from build123d import *

# Parameters (mm, degrees)
F0_W     = 50
F0_H     = 50
F1_DEPTH = 35
F3_DEPTH = 35.001
F5_DEPTH = 20


with BuildPart() as f1:
    # F0 (on Front) → F1 (new body)
    with BuildSketch(Plane.XZ):
        Rectangle(F0_W, F0_H)
    extrude(amount=F1_DEPTH)

    # F2 (on face) → F3 (cut, through all)
    with BuildSketch(Plane.XZ.offset(35)):
        Polygon((-25, 0), (18.30127, 25), (-25, 25), align=None)
    extrude(amount=-F3_DEPTH, mode=Mode.SUBTRACT)

    # F4 (on face) → F5 (cut)
    with BuildSketch(Plane.XZ.offset(35)):
        Polygon((-25, 0), (-25, -13), (25, -13), (25, 13), (-2.48334, 13), align=None)
    extrude(amount=-F5_DEPTH, mode=Mode.SUBTRACT)


solid = f1.part
Could you check a few things on this model? Use its own coordinates, in mm. A direction names the side the tool comes from. Give positions to 0.01 mm unless a question says otherwise; leave off trailing zeros. Write each loop counter-clockwise with the first axis right and the second up, starting at its lowest first coordinate (ties: lowest second). Pieces come first, ordered by that corner, then holes. Notation, with made-up numbers: (-3.75, 15.25) -> (26.25, 15.25) arc R5 ccw to (26.25, 21.25) -> close; hole circle Ø5 at (48.25, -30.5). An arc over 180 degrees is marked (long way). Write each question's results on one line, items separated by ' | '. Start each with the question number.
Q1. I'm going to push flat-ended pins straight in: pin 1 Ø2 at (x, y) = (-12.5, -31) entering from +Z; pin 2 Ø6 at (x, z) = (2.5, 4) entering from -Y; pin 3 Ø2 at (y, z) = (-20.5, 16.5) entering from -X. Where does each tip first touch, or does it pass through?
Q2. Suppose I cut it at A-A, the plane y = -20.5. List the corners of the cut face in (x, z) for me, and give its area (3 significant figures).
Q3. I need wall thicknesses on probe 1 along Z at (x, y) = (20, -18); probe 2 along Z at (x, y) = (-18.5, -27); probe 3 along Y at (x, z) = (19, 3). Which ranges of each line are inside material? Lowest first, please.
Q4. Suppose I cut it at D-D, the plane z = 21. List the corners of the cut face in (x, y) for me, and give its area (3 significant figures).
Q5. Suppose I cut it at C-C, the plane y = -11.5. List the corners of the cut face in (x, z) for me.
Q6. Suppose I cut it at B-B, the plane x = 20. List the corners of the cut face in (y, z) for me.
Q7. We'd pull the mould along Z, two halves only. Please class faces 3 (the face through (0, -25, -13)), 4 (the face through (1.159, -13.856, 15.103)), 5 (the face through (-25, -13, -15)): +Z half, -Z half, draft (parallel to the pull), parting line (faces both ways), or undercut.
Q8. Which directions (+Z, -Z, +X, -X, +Y, -Y) give clear straight access to the entire face, cutting with the end or side of a thin tool? Please do faces 1 (the face through (0, -15, 0)), 2 (the face through (0, -35, -19)).
Outcome:
1) pin 1: z = -13 | pin 2: y = -15 | pin 3: x = 1.85
2) outline: (-25, -25) -> (25, -25) -> (25, -13) -> (-25, -13) -> close; (-2.48, 13) -> (25, 13) -> (25, 25) -> (18.3, 25) -> close | area: 805 mm2
3) probe 1: -25 to -13, 13 to 25 | probe 2: -25 to -13 | probe 3: -15 to 0
4) outline: (11.37, -35) -> (25, -35) -> (25, 0) -> (11.37, 0) -> close | area: 477 mm2
5) outline: (-25, -25) -> (25, -25) -> (25, 25) -> (18.3, 25) -> (-25, 0) -> close
6) outline: (-35, -25) -> (0, -25) -> (0, 25) -> (-35, 25) -> (-35, 13) -> (-15, 13) -> (-15, -13) -> (-35, -13) -> close
7) face 3: undercut | face 4: +Z half | face 5: draft
8) face 1: +X, -X, -Y | face 2: +Z, -Z, +X, -X, -Y
